Can you work these out from the model? Positions are in its coordinate system, mm. A direction names the side the tool comes from. Coordinates: 2 decimals unless noted, no trailing zeros. Loops run counter-clockwise (first coordinate to the right, second up) from the corner with the lowest first, then second, coordinate; pieces in that order, holes last. Notation, with made-up numbers: (20.5, 45) -> (35.5, 45) arc R19 cw to (35.5, 72) -> close; hole circle Ø8 at (18.25, -29.75). An arc over 180 degrees is marked (long way). Use one line per item in the form item = value. Start each with the question number.
(1) Imagine slicing it at B-B (x = 5). List the corners of the cut face in (y, z) for me, plus the area to 3 significant figures.
(2) Imagine slicing it at C-C (z = -82). List the corners of the cut face in (x, y) for me.
(3) I'm going to push flat-ended pins straight in: pin 1 (1 mm diameter, centred on x = 4.5, z = -23, fed in from +Y); pin 2 (1.5 mm diameter, centred on y = 58.5, z = -104.5, fed in from -X); pin 3 (3 mm diameter, centred on y = 57, z = -56, fed in from +X). Where does each tip first touch, or does it pass through?
(4) Imagine slicing it at A-A (y = 60). List the corners of the cut face in (x, z) for me.
(5) On a 3-axis mill with a long thin cutter (end or side, diameter ignored), from which of +Z, -Z, +X, -X, +Y, -Y can I reach the whole of each face in a straight line? I mean faces 1 (the flat face through (5, 60, -120)), 2 (the cylindrical face through (4.577, 56.778, -60.84)). Say none if no direction works.
(6) I need wall thicknesses on line 1 (Y direction, x = 4.75, z = -89.5); line 2 (Y direction, x = 7, z = -37); line 3 (Z direction, x = 6, y = 64.25). Which ranges of each line are inside material? Lowest first, please. Write a range as [from, to].
```python
from build123d import *

# Parameters (mm, degrees)
SKETCH1_R           = 3.25
SKETCH3_R           = 5
BOSS_EXTRUDE1_DEPTH = 3
DOME1_FACE_RADIUS   = 5
DOME1_HEIGHT        = 3


with BuildPart() as part:
    # Sweep1: sweep along a path in Sketch2
    with BuildLine(Plane(origin=(5, 0, 0), x_dir=(0, 0, -1), z_dir=(1, 0, 0))) as sweep1_path:
        Line((0, 0), (120, 0))
    # Sketch1 → Sweep1 (sweep)
    with BuildSketch(Plane.XY):
        with Locations((5, 60)):
            Circle(SKETCH1_R)
    sweep(path=sweep1_path.line)

    # Sketch3 → Boss-Extrude1 (add)
    with BuildSketch(Plane.XY):
        with Locations((5, 60)):
            Circle(SKETCH3_R)
    extrude(amount=BOSS_EXTRUDE1_DEPTH)

    # Dome1: a dome of height H over a round flat face of radius A is a cap of a sphere of radius (A * A + H * H) / (2 * H)
    dome1_r = (DOME1_FACE_RADIUS * DOME1_FACE_RADIUS + DOME1_HEIGHT * DOME1_HEIGHT) / (2 * DOME1_HEIGHT)
    dome1_base = Plane((5, 60, 3), z_dir=(0, 0, 1))
    with Locations(dome1_base.offset(DOME1_HEIGHT - dome1_r)):
        dome1_ball = Sphere(dome1_r, mode=Mode.PRIVATE)
    add(split(dome1_ball, bisect_by=dome1_base, keep=Keep.TOP, mode=Mode.PRIVATE))


solid = part.part
```
Worked out:
q1.outline = (55, 0) -> (56.75, 0) -> (56.75, -120) -> (63.25, -120) -> (63.25, 0) -> (65, 0) -> (65, 3) arc R5.67 ccw to (55, 3) -> close
q1.area = 831 mm2
q2.outline = circle Ø6.5 at (5, 60)
q3.pin_1 = 63.25
q3.pin_2 = 1.84
q3.pin_3 = 7.88
q4.outline = (0, 0) -> (1.75, 0) -> (1.75, -120) -> (8.25, -120) -> (8.25, 0) -> (10, 0) -> (10, 3) arc R5.67 ccw to (0, 3) -> close
q5.face_1 = -Z, +X, -X, +Y, -Y
q5.face_2 = -Z
q6.line_1 = [56.76, 63.24]
q6.line_2 = [57.44, 62.56]
q6.line_3 = [0, 3.95]
